Model file for the job. Use its own axes, mm. A direction names the side the tool comes from. Coordinates: 2 decimals unless noted, no trailing zeros. Write each loop counter-clockwise with the first axis right and the second up, starting at its lowest first coordinate (ties: lowest second). Pieces come first, ordered by that corner, then holes. Notation, with made-up numbers: (79, -30) - (94, -30) arc R22 ccw to (94, -4) - close; hole circle Ø11 at (20, -33.75). An arc over 180 degrees is marked (long way). Put each result on its own line as item: value. Start each with the question number.
1. Drill centre lines: L1, parallel to X at y = 6.35, z = -23.25 (3 decimals); L2, parallel to X at y = 6.25, z = 0; L3, parallel to Z at x = 41, y = 5.25 (3 decimals). Where is each one in solid material? Low to high. Write a range as from..to.
2. Saw through at D-D, the plane z = 11.5. Give the number of separate pieces and of enclosed holes in the cut face, plus the area to 3 significant figures.
3. Saw through at C-C, the plane y = 3.75. Write the cut outline in (x, z) (3 decimals), plus the area to 3 significant figures.
4. Saw through at B-B, the plane x = 6. Write the cut outline in (y, z) (3 decimals).
5. Saw through at A-A, the plane y = 9.5. Write the cut outline in (x, z) (3 decimals), plus the area to 3 significant figures.
6. Pull direction Z, two halves, no side cores. Call faces 3 (the face through (22, 6, -25.4)), 4 (the face through (44.45, 6, 22)), 5 (the face through (1.261, 9, -19)): released by +Z, released by -Z, zero draft, split by the parting line, or undercut.
7. Which spindle directions (+Z, -Z, +X, -X, +Y, -Y) get a long thin tool onto all of the face, cutting with end or side? Do faces 1 (the face through (37.77, 6.43, -0.22)), 2 (the face through (7.7, 4.8, -19.1)). Say none if no direction does.
8. Drop flat-ended pins along their axis: P1, Ø1.9, axis at y = 9, z = -18, coming from the +X side; P2, Ø2, axis at x = 39.52, y = 6.35, coming from the +Z side; P3, Ø2, axis at y = 11, z = -7, coming from the +X side. Give the stop position or say it passes through.
```python
from build123d import *

# Parameters (mm, degrees)
SKETCH1_W           = 44.45
SKETCH1_H           = 12.7
SKETCH1_R           = 1.7526
BOSS_EXTRUDE1_DEPTH = 25.4
CUT_EXTRUDE1_START  = -3.175
CUT_EXTRUDE1_DEPTH  = 6.35
CUT_EXTRUDE2_START  = -47.625
CUT_EXTRUDE2_DEPTH  = 6.35
CUT_EXTRUDE3_DEPTH  = 53.74706153
FILLET1_ANGLE       = 7.76917
FILLET1_2_ANGLE     = 7.76917
FILLET1_3_ANGLE     = 7.76917
FILLET1_4_ANGLE     = 7.76917


with BuildPart() as part:
    # Sketch1 → Boss-Extrude1 (new, symmetric)
    with BuildSketch(Plane.XY):
        with Locations((22.225, 6.35)):
            Rectangle(SKETCH1_W, SKETCH1_H)
        with Locations((4.9276, 6.35)):
            Circle(SKETCH1_R, mode=Mode.SUBTRACT)
        with Locations((39.5224, 6.35)):
            Circle(SKETCH1_R, mode=Mode.SUBTRACT)
    extrude(amount=BOSS_EXTRUDE1_DEPTH, both=True)

    # Sketch2 → Cut-Extrude1 (cut)
    with BuildSketch(Plane.XY.offset(25.4).offset(CUT_EXTRUDE1_START)):
        Polygon((1.261425791, 6.35), (1.261425791, 14.915819411), (8.593774209, 14.915819411), (8.593774209, 6.35), (6.760687105, 3.175), (3.094512895, 3.175), align=None)
        Polygon((35.856225791, 6.35), (37.689312895, 3.175), (41.355487105, 3.175), (43.188574209, 6.35), (43.188574209, 16.066451869), (35.856225791, 16.066451869), align=None)
    extrude(amount=-CUT_EXTRUDE1_DEPTH, mode=Mode.SUBTRACT)

    # Sketch2<2> → Cut-Extrude2 (cut)
    with BuildSketch(Plane.XY.offset(25.4).offset(CUT_EXTRUDE2_START)):
        Polygon((1.261425791, 6.35), (1.261425791, 14.915819411), (8.593774209, 14.915819411), (8.593774209, 6.35), (6.760687105, 3.175), (3.094512895, 3.175), align=None)
        Polygon((35.856225791, 6.35), (37.689312895, 3.175), (41.355487105, 3.175), (43.188574209, 6.35), (43.188574209, 16.066451869), (35.856225791, 16.066451869), align=None)
    extrude(amount=CUT_EXTRUDE2_DEPTH, mode=Mode.SUBTRACT)

    # Sketch3 → Cut-Extrude3 (cut, through all)
    with BuildSketch(Plane.XZ):
        with BuildLine():
            Line((44.45, 19.05), (44.45, -19.05))
            ThreePointArc((44.45, -19.05), (43.965232978, 0), (44.45, 19.05))
        make_face()
        with BuildLine():
            Line((0, 19.05), (0, -19.05))
            ThreePointArc((0, -19.05), (0.484767022, 0), (0, 19.05))
        make_face()
    extrude(amount=-CUT_EXTRUDE3_DEPTH, mode=Mode.SUBTRACT)

    # Fillet1: read off the stored shape, not the designer's step
    # Fillet1 outline → Fillet1 (revolve, cut)
    with BuildSketch(Plane(origin=(418.513709618, 0, 0), x_dir=(-0.9977025418167154, 0, -0.0677468674734517), z_dir=(0.0677468674734517, 0, -0.9977025418167154))):
        with BuildLine():
            Line((374.54847664, 12.7), (374.54847664, 12.065))
            ThreePointArc((374.54847664, 12.065), (374.734463834, 12.514012806), (375.18347664, 12.7))
            Line((375.18347664, 12.7), (374.54847664, 12.7))
        make_face()
    revolve(axis=Axis((418.513709618, 0, 0), (0, 1, 0)), revolution_arc=FILLET1_ANGLE, mode=Mode.SUBTRACT)

    # Fillet1 2 outline → Fillet1 2 (revolve, cut)
    with BuildSketch(Plane(origin=(418.513709618, 0, 0), x_dir=(-0.9977025418167154, 0, -0.0677468674734517), z_dir=(0.0677468674734517, 0, -0.9977025418167154))):
        with BuildLine():
            ThreePointArc((375.18347664, 0), (374.734463834, 0.185987194), (374.54847664, 0.635))
            Line((374.54847664, 0.635), (374.54847664, 0))
            Line((374.54847664, 0), (375.18347664, 0))
        make_face()
    revolve(axis=Axis((418.513709618, 0, 0), (0, 1, 0)), revolution_arc=FILLET1_2_ANGLE, mode=Mode.SUBTRACT)

    # Fillet1 3 outline → Fillet1 3 (revolve, cut)
    with BuildSketch(Plane(origin=(-374.063709618, 0, 0), x_dir=(0.9977025418167152, 0, 0.06774686747345202), z_dir=(-0.06774686747345202, 0, 0.9977025418167152))):
        with BuildLine():
            Line((374.54847664, 12.7), (374.54847664, 12.065))
            ThreePointArc((374.54847664, 12.065), (374.734463834, 12.514012806), (375.18347664, 12.7))
            Line((375.18347664, 12.7), (374.54847664, 12.7))
        make_face()
    revolve(axis=Axis((-374.063709618, 0, 0), (0, 1, 0)), revolution_arc=FILLET1_3_ANGLE, mode=Mode.SUBTRACT)

    # Fillet1 4 outline → Fillet1 4 (revolve, cut)
    with BuildSketch(Plane(origin=(-374.063709618, 0, 0), x_dir=(0.9977025418167152, 0, 0.06774686747345202), z_dir=(-0.06774686747345202, 0, 0.9977025418167152))):
        with BuildLine():
            ThreePointArc((375.18347664, 0), (374.734463834, 0.185987194), (374.54847664, 0.635))
            Line((374.54847664, 0.635), (374.54847664, 0))
            Line((374.54847664, 0), (375.18347664, 0))
        make_face()
    revolve(axis=Axis((-374.063709618, 0, 0), (0, 1, 0)), revolution_arc=FILLET1_4_ANGLE, mode=Mode.SUBTRACT)


solid = part.part
```
Final values:
1. L1: x = 0..3.175, 6.68..37.77, 41.275..44.45
1. L2: x = 0.48..3.18, 6.68..37.77, 41.27..43.97
1. L3: z = -25.4..-22.225, -15.875..15.875, 22.225..25.4
2. separate pieces: 1
2. enclosed holes: 2
2. area: 537 mm²
3. outline: (0, -25.4) - (44.45, -25.4) - (44.45, -19.05) arc R374.548 cw to (44.45, 19.05) - (44.45, 25.4) - (0, 25.4) - (0, 19.05) arc R374.548 cw to (0, -19.05) - close; hole (2.763, -22.225) - (7.093, -22.225) - (7.093, -15.875) - (2.763, -15.875) - close; hole (2.763, 15.875) - (7.093, 15.875) - (7.093, 22.225) - (2.763, 22.225) - close; hole (37.357, -22.225) - (41.687, -22.225) - (41.687, -15.875) - (37.357, -15.875) - close; hole (37.357, 15.875) - (41.687, 15.875) - (41.687, 22.225) - (37.357, 22.225) - close
3. area: 2,120 mm²
4. outline: (0, -25.4) - (4.964, -25.4) - (4.964, -22.225) - (3.175, -22.225) - (3.175, -15.875) - (4.964, -15.875) - (4.964, 15.875) - (3.175, 15.875) - (3.175, 22.225) - (4.964, 22.225) - (4.964, 25.4) - (0, 25.4) - close; (7.736, -25.4) - (12.7, -25.4) - (12.7, -22.225) - (7.736, -22.225) - close; (7.736, -15.875) - (12.7, -15.875) - (12.7, 15.875) - (7.736, 15.875) - close; (7.736, 22.225) - (12.7, 22.225) - (12.7, 25.4) - (7.736, 25.4) - close
5. outline: (0, -25.4) - (44.45, -25.4) - (44.45, -19.05) arc R374.548 cw to (44.45, 19.05) - (44.45, 25.4) - (0, 25.4) - (0, 19.05) arc R374.548 cw to (0, -19.05) - close; hole (1.261, -22.225) - (8.594, -22.225) - (8.594, -15.875) - (1.261, -15.875) - close; hole (1.261, 15.875) - (8.594, 15.875) - (8.594, 22.225) - (1.261, 22.225) - close; hole (35.856, -22.225) - (43.189, -22.225) - (43.189, -15.875) - (35.856, -15.875) - close; hole (35.856, 15.875) - (43.189, 15.875) - (43.189, 22.225) - (35.856, 22.225) - close
5. area: 2,050 mm²
6. face 3: released by -Z
6. face 4: zero draft
6. face 5: undercut
7. face 1: +Z, -Z
7. face 2: +Y
8. P1: stops at x = 44.44
8. P2: passes through
8. P3: stops at x = 44.05
